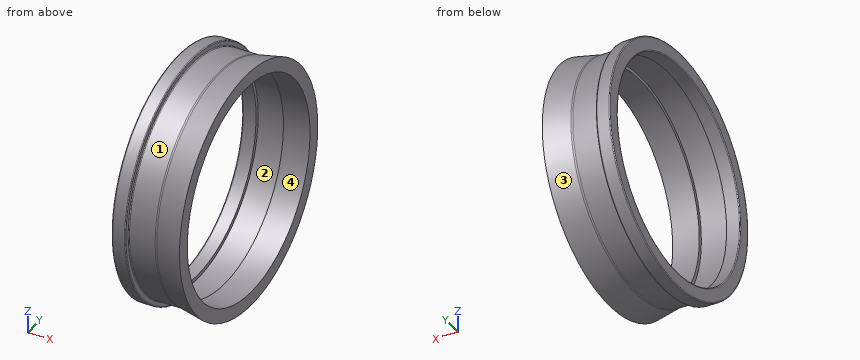
from build123d import *

# Parameters (mm, degrees)
F3_R     = 50
F4_R     = 5
F5_W     = 906.862557
F5_H     = 1744.742334
F6_DEPTH = 1000


with BuildPart() as f2:
    # F0 (on Front) → F2 (revolve)
    with BuildSketch(Plane.XZ):
        Polygon((75, 660), (0, 660), (0, 585), (75, 585), (75, 605), (225, 605), (225, 585), (1070, 585), (1070, 685), (500, 685), (225, 630), (75, 630), align=None)
    revolve(axis=Axis((388.548315, 0, 0), (1, 0, 0)))

    # F3
    f3_edges = [f2.edges().sort_by_distance(p)[0] for p in [
        (500, 0, -685),
        (225, 0, -630),
    ]]
    fillet(f3_edges, radius=F3_R)

    # F4
    f4_edges = [f2.edges().sort_by_distance(p)[0] for p in [
        (75, 0, -660),
        (75, 0, -630),
        (0, 0, -660),
        (0, 0, -585),
        (1070, 0, -685),
    ]]
    fillet(f4_edges, radius=F4_R)

    # F5 (on Front) → F6 (cut, symmetric)
    with BuildSketch(Plane.XZ):
        with Locations((824.053854, 4.612178)):
            Rectangle(F5_W, F5_H)
    extrude(amount=F6_DEPTH, both=True, mode=Mode.SUBTRACT)


solid = f2.part
Can you work these out from the model? Positions are in its coordinate system, mm. Face numbers are marked on the shaded views. A direction names the side the tool comes from. Coordinates: 2 decimals unless noted, no trailing zeros. Loops run counter-clockwise (first coordinate to the right, second up) from the corner with the lowest first, then second, coordinate; pieces in that order, holes last. Notation, with made-up numbers: M 44,56.5 L 86,56.5 A8 ccw 86,61.5 Z; hole C -29.75,-37 d5. An arc over 180 degrees is marked long. Return JSON: item names as keys, results as strings. Group by question number.
Item 1: On a 3-axis mill with a long thin cutter (end or side, diameter ignored), from which of +Z, -Z, +X, -X, +Y, -Y can I reach the whole of each face in a straight line? I mean the marked faces 3 and 4. Say none if no direction works.
Item 2: I'm going to push flat-ended pins straight in: pin 1 Ø3 at (x, y) = (171, -159.5) entering from -Z; pin 2 Ø3 at (x, y) = (113.5, 265) entering from -Z; pin 3 Ø3 at (x, y) = (306, -401.5) entering from +Z. Where does each tip first touch, or does it pass through?
Item 3: Imagine slicing it at B-B (x = 112). Please give me the cut outline in (y, z).
Item 4: If I drill on L1, parallel to Y at x = 39, z = 0; L2, parallel to Y at x = 165, z = 0; L3, parallel to Z at x = 169.5, y = -14.5, over which ranges is the centre line in solid material (lowest first)? Write a range as from..to.
Item 5: Imagine slicing it at A-A (x = 313.5). Please give me the cut outline in (y, z), and give its area (3 significant figures).
Item 6: Thinking about a two-plate mould opening in Y: for the marked faces 1 and 2, which applies, released by +Y, released by -Y, zero draft, split by the parting line, or undercut?
Verdict:
{
 "1": {"face 3": "none", "face 4": "+X, -X"},
 "2": {"pin 1": "stops at z = -609.87", "pin 2": "stops at z = -572.25", "pin 3": "stops at z = 507.58"},
 "3": {"outline": "C 0,0 d1260; hole C 0,0 d1210"},
 "4": {"L1": "y = -660..-585, 585..660", "L2": "y = -630..-605, 605..630", "L3": "z = -629.83..-604.83, 604.83..629.83"},
 "5": {"outline": "C 0,0 d1295.4; hole C 0,0 d1170", "area": "243,000 mm^2"},
 "6": {"face 1": "split by the parting line", "face 2": "undercut"}
}
